For this review, take the finished solid that the model builds, in its own axes (mm). Face numbers are marked on the shaded views. Coordinates: 2 decimals unless noted, no trailing zeros. Loops run counter-clockwise (first coordinate to the right, second up) from the corner with the lowest first, then second, coordinate; pieces in that order, holes last. Notation, with made-up numbers: (-29, 20.25) - (6, 20.25) arc R23 ccw to (6, 40.25) - close; hole circle Ø11 at (5, 71.5). An arc over 180 degrees is marked (long way). Use one line per item in the form item = value. Start each with the question number.
1. To check wall thickness, follow probe 1 along X at (y, z) = (2.8, 0); probe 2 along X at (y, z) = (3.6, 0.75); probe 3 along X at (y, z) = (5.2, 5). State the ranges of each line that lie inside material, in increasing order.
2. Add section A-A on x = 27.5. Give the boundary of the cut face in (y, z), and give its area (3 significant figures).
3. Add section B-B on z = 0. Give the boundary of the cut face in (x, y).
4. Add section C-C on y = 1. Give the boundary of the cut face in (x, z).
5. Add section D-D on x = 15.5. Give the boundary of the cut face in (y, z).
6. Draft analysis for pull direction X (two halves, no side actions). For the marked faces 1, 2 and 3, state which applies: +X half, -X half, draft (parallel to the pull), parting line (faces both ways), or undercut.
7. For pin 1 Ø2 at (x, z) = (-15.5, 0) entering from +Y; pin 2 Ø3 at (y, z) = (2.5, -4.5) entering from -X, all flat-tipped, find the tip position at first contact; note any pin that passes through.
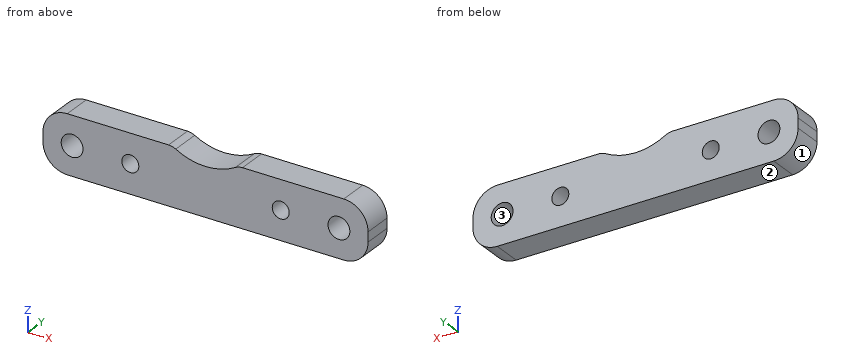
```python
from build123d import *

# Parameters (mm, degrees)
SKETCH1_R           = 1.75
SKETCH1_R_2         = 2.25
BOSS_EXTRUDE1_DEPTH = 6


with BuildPart() as part:
    # Sketch1 → Boss-Extrude1 (new body)
    with BuildSketch(Plane(origin=(0, 0, 0), x_dir=(1, 0, 0), z_dir=(0, 1, 0))):
        with BuildLine():
            Line((-28.5, 6), (28.5, 6))
            ThreePointArc((28.5, 6), (32.035533906, 4.535533906), (33.5, 1))
            Line((33.5, 1), (33.5, -1))
            ThreePointArc((33.5, -1), (32.035533906, -4.535533906), (28.5, -6))
            Line((28.5, -6), (7.615773106, -6))
            ThreePointArc((7.615773106, -6), (6.853772344, -5.901612455), (6.141752505, -5.612903226))
            ThreePointArc((6.141752505, -5.612903226), (0, -4), (-6.141752505, -5.612903226))
            ThreePointArc((-6.141752505, -5.612903226), (-6.853772344, -5.901612455), (-7.615773106, -6))
            Line((-7.615773106, -6), (-28.5, -6))
            ThreePointArc((-28.5, -6), (-32.035533906, -4.535533906), (-33.5, -1))
            Line((-33.5, -1), (-33.5, 1))
            ThreePointArc((-33.5, 1), (-32.035533906, 4.535533906), (-28.5, 6))
        make_face()
        with Locations(Location((-15.5, 0, 0), (0, 0, 270))):
            Circle(SKETCH1_R, mode=Mode.SUBTRACT)
        with Locations(Location((15.5, 0, 0), (0, 0, 270))):
            Circle(SKETCH1_R, mode=Mode.SUBTRACT)
        with Locations(Location((27.5, 0, 0), (0, 0, 270))):
            Circle(SKETCH1_R_2, mode=Mode.SUBTRACT)
        with Locations(Location((-27.5, 0, 0), (0, 0, 270))):
            Circle(SKETCH1_R_2, mode=Mode.SUBTRACT)
    extrude(amount=BOSS_EXTRUDE1_DEPTH)


solid = part.part
```
Conclusion:
q1.probe_1 = -33.5 to -29.75, -25.25 to -17.25, -13.75 to 13.75, 17.25 to 25.25, 29.75 to 33.5
q1.probe_2 = -33.5 to -29.62, -25.38 to -17.08, -13.92 to 13.92, 17.08 to 25.38, 29.62 to 33.5
q1.probe_3 = -31.5 to -4.9, 4.9 to 31.5
q2.outline = (0, -6) - (6, -6) - (6, -2.25) - (0, -2.25) - close; (0, 2.25) - (6, 2.25) - (6, 6) - (0, 6) - close
q2.area = 45.0 mm^2
q3.outline = (-33.5, 0) - (-29.75, 0) - (-29.75, 6) - (-33.5, 6) - close; (-25.25, 0) - (-17.25, 0) - (-17.25, 6) - (-25.25, 6) - close; (-13.75, 0) - (13.75, 0) - (13.75, 6) - (-13.75, 6) - close; (17.25, 0) - (25.25, 0) - (25.25, 6) - (17.25, 6) - close; (29.75, 0) - (33.5, 0) - (33.5, 6) - (29.75, 6) - close
q4.outline = (-33.5, -1) arc R5 ccw to (-28.5, -6) - (28.5, -6) arc R5 ccw to (33.5, -1) - (33.5, 1) arc R5 ccw to (28.5, 6) - (7.62, 6) arc R3 ccw to (6.14, 5.61) arc R12.5 cw to (-6.14, 5.61) arc R3 ccw to (-7.62, 6) - (-28.5, 6) arc R5 ccw to (-33.5, 1) - close; hole circle Ø4.5 at (-27.5, 0); hole circle Ø3.5 at (-15.5, 0); hole circle Ø3.5 at (15.5, 0); hole circle Ø4.5 at (27.5, 0)
q5.outline = (0, -6) - (6, -6) - (6, -1.75) - (0, -1.75) - close; (0, 1.75) - (6, 1.75) - (6, 6) - (0, 6) - close
q6.face_1 = -X half
q6.face_2 = draft
q6.face_3 = undercut
q7.pin_1 = through
q7.pin_2 = -33.08
